from build123d import *

# Parameters (mm, degrees)
EXTRUDE_THIN1_DEPTH = 9.525
EXTRUDE_THIN2_DEPTH = 4.445
SKETCH3_R           = 2.3749
SKETCH3_R_2         = 0.7874
CUT_EXTRUDE1_DEPTH  = 24.37151185


with BuildPart() as part:
    # Sketch1 → Extrude-Thin1 (new body)
    with BuildSketch(Plane.XY):
        with BuildLine():
            Line((6.7437, 17.77238356), (6.368570529, 16.208915196))
            ThreePointArc((6.368570529, 16.208915196), (9.034076329, 9.242376411), (5.5626, 2.640373995))
            Line((5.5626, 2.640373995), (5.5626, 0))
            Line((5.5626, 0), (-5.5626, 0))
            Line((-5.5626, 0), (-5.5626, 2.640373995))
            ThreePointArc((-5.5626, 2.640373995), (-9.034076329, 9.242376411), (-6.368570529, 16.208915196))
            Line((-6.368570529, 16.208915196), (-6.7437, 17.77238356))
            Line((-6.7437, 17.77238356), (-7.040088077, 17.701269935))
            Line((-7.040088077, 17.701269935), (-6.704567446, 16.30288369))
            ThreePointArc((-6.704567446, 16.30288369), (-9.337658307, 9.212943132), (-5.8674, 2.492992844))
            Line((-5.8674, 2.492992844), (-5.8674, -0.3048))
            Line((-5.8674, -0.3048), (5.8674, -0.3048))
            Line((5.8674, -0.3048), (5.8674, 2.492992844))
            ThreePointArc((5.8674, 2.492992844), (9.337658307, 9.212943132), (6.704567446, 16.30288369))
            Line((6.704567446, 16.30288369), (7.040088077, 17.701269935))
            Line((7.040088077, 17.701269935), (6.7437, 17.77238356))
        make_face()
    extrude(amount=EXTRUDE_THIN1_DEPTH)

    # Sketch2 → Extrude-Thin2 (add, symmetric)
    with BuildSketch(Plane(origin=(0, 0, 0), x_dir=(0, 0, -1), z_dir=(1, 0, 0))):
        Polygon((0, 0), (3.6068, 0), (0.650543656, 13.916451143), (1.950898512, 16.503333624), (2.223228171, 16.366440976), (0.970920321, 13.875141604), (3.983149653, -0.3048), (0, -0.3048), align=None)
    extrude(amount=EXTRUDE_THIN2_DEPTH, both=True)

    # Sketch3 → Cut-Extrude1 (cut, through all)
    with BuildSketch(Plane(origin=(0, 0.733106356, -3.451067026), x_dir=(1, 0, 0), z_dir=(0, -0.2077922077922076, 0.9781729900078207))):
        with Locations(Location((0, 9.029535065, 0), (0, 0, 270))):
            Circle(SKETCH3_R)
        with Locations(Location((2.89696051, 3.586960276, 0), (0, 0, 270))):
            Circle(SKETCH3_R_2)
    extrude(amount=-CUT_EXTRUDE1_DEPTH, mode=Mode.SUBTRACT)

    # Sketch4 → Revolve2 (revolve)
    with BuildSketch(Plane(origin=(0, 0, 0), x_dir=(0, 0, -1), z_dir=(1, 0, 0))):
        with BuildLine():
            Line((0.034373175, 9.2383225), (0.305728617, 9.295966237))
            ThreePointArc((0.305728617, 9.295966237), (0.288117278, 10.713567235), (1.081314286, 11.888616703))
            Line((1.081314286, 11.888616703), (1.017979221, 12.186763831))
            ThreePointArc((1.017979221, 12.186763831), (0.048720075, 10.871823503), (0.034373175, 9.2383225))
        make_face()
    revolve(axis=Axis((0, 9.2383225, -0.034373175), (0, 0.20779220779220853, -0.9781729900078205)))


solid = part.part
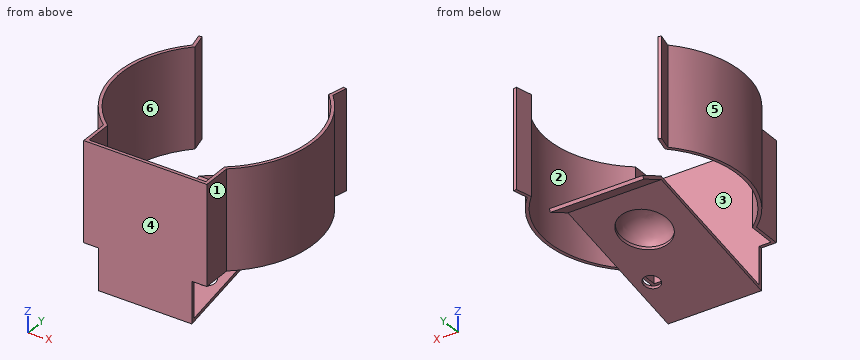
CAD build for the part. Positions are in the model's coordinates, mm. Face numbers are marked on the shaded views. A direction names the side the tool comes from. Round coordinates to 2 decimals unless told otherwise and drop trailing zeros. Write each loop counter-clockwise with the first axis right and the second up, starting at its lowest first coordinate (ties: lowest second). Pieces come first, ordered by that corner, then holes.
(1) Slice it at B-B, the plane x = -3.75. Write the cut outline in (y, z) (3 decimals), and give its area (3 significant figures).
(2) Drop flat-ended pins along their axis: P1, Ø2, axis at y = 10, z = -1.5, coming from the +X side (3 decimals); P2, Ø0.8, axis at y = 0.5, z = 3, coming from the +X side; P3, Ø3, axis at y = 1.5, z = 5, coming from the +X side. Give the stop position or say it passes through.
(3) Probe line 1 along X through (y, z) = (2, 2.5); line 2 along Y through (x, z) = (5, 8.25); line 3 along X through (y, z) = (14, -0.75) (3 decimals). List the from-to ranges inside material, lowest first.
(4) Slice it at D-D, the plane y = 12.5. Write the cut outline in (x, z) (3 decimals), and give its area (3 significant figures).
(5) 3-axis set-ups, long thin cutter, end or side, ignore diameter. For the marked faces 1, 2 and 3: which of +Z, -Z, +X, -X, +Y, -Y reach the whole face in a straight line?
(6) Mould opens along X. For the marked faces 4, 5 and 6 say: pulls with the +X half, pulls with the -X half, needs draft (parallel to the pull), parting line crosses it, or undercut.
(7) Slice it at C-C, the plane z = 7.5. Write the cut outline in (x, y), and give its area (3 significant figures).
(8) Slice it at A-A, the plane y = 15.75. Write the cut outline in (x, z) (3 decimals), and give its area (3 significant figures).
From the geometry:
1. outline: (-0.305, -3.983) - (13.875, -0.971) - (16.366, -2.223) - (16.503, -1.951) - (13.916, -0.651) - (0, -3.607) - (0, 9.525) - (-0.305, 9.525) - close
1. area: 9.30 mm2
2. P1: stops at x = 4.445
2. P2: stops at x = 5.87
2. P3: stops at x = 6.45
3. line 1: x = -5.87 to -5.56, 5.56 to 5.87
3. line 2: y = -0.3 to 0
3. line 3: x = -4.445 to 4.445
4. outline: (-8.95, 0) - (-8.631, 0) - (-8.631, 9.525) - (-8.95, 9.525) - close; (-4.445, -1.263) - (4.445, -1.263) - (4.445, -0.951) - (-4.445, -0.951) - close; (8.631, 0) - (8.95, 0) - (8.95, 9.525) - (8.631, 9.525) - close
4. area: 8.85 mm2
5. face 1: +Z, -Z, +X, -Y
5. face 2: +Z, -Z
5. face 3: +Z
6. face 4: needs draft
6. face 5: pulls with the -X half
6. face 6: undercut
7. outline: (-7.04, 17.7) - (-6.7, 16.3) arc R9.35 ccw to (-5.87, 2.49) - (-5.87, -0.3) - (5.87, -0.3) - (5.87, 2.49) arc R9.35 ccw to (6.7, 16.3) - (7.04, 17.7) - (6.74, 17.77) - (6.37, 16.21) arc R9.05 cw to (5.56, 2.64) - (5.56, 0) - (-5.56, 0) - (-5.56, 2.64) arc R9.05 cw to (-6.37, 16.21) - (-6.74, 17.77) - close
7. area: 15.5 mm2
8. outline: (-7.201, 0) - (-6.801, 0) - (-6.801, 9.525) - (-7.201, 9.525) - close; (-4.445, -1.913) - (4.445, -1.913) - (4.445, -1.572) - (-4.445, -1.572) - close; (6.801, 0) - (7.201, 0) - (7.201, 9.525) - (6.801, 9.525) - close
8. area: 10.7 mm2
